Read the model definition and answer for the solid it produces. Units are mm, in the model's axes. A direction names the side the tool comes from. Coordinates: 2 decimals unless noted, no trailing zeros. Loops run counter-clockwise (first coordinate to the right, second up) from the corner with the lowest first, then second, coordinate; pieces in that order, holes last.
from build123d import *

# Parameters (mm, degrees)
SKETCH1_R               = 23
BOSS_EXTRUDE3_DEPTH     = 10
SKETCH3_R               = 23
SKETCH3_R_2             = 13
CUT_EXTRUDE1_DEPTH      = 4
SKETCH4_R               = 1.725
SKETCH4_R_2             = 2.725
CUT_EXTRUDE2_DEPTH      = 35.029399054
SKETCH5_R               = 6.5
CUT_EXTRUDE3_DEPTH      = 5
SKETCH6_R               = 2.725
CUT_EXTRUDE4_DEPTH      = 35.029399054
CUT_EXTRUDE5_DEPTH      = 34.075670817
CUT_EXTRUDE5_DEPTH_BACK = 4
FILLET1_R               = 2


with BuildPart() as part:
    # Sketch1 → Boss-Extrude3 (new body)
    with BuildSketch(Plane.XY):
        Circle(SKETCH1_R)
    extrude(amount=BOSS_EXTRUDE3_DEPTH)

    # Sketch3 → Cut-Extrude1 (cut)
    with BuildSketch(Plane(origin=(0, 0, 0), x_dir=(-1, 0, 0), z_dir=(0, 0, -1))):
        Circle(SKETCH3_R)
        Circle(SKETCH3_R_2, mode=Mode.SUBTRACT)
    extrude(amount=-CUT_EXTRUDE1_DEPTH, mode=Mode.SUBTRACT)

    # Sketch4 → Cut-Extrude2 (cut, through all)
    with BuildSketch(Plane(origin=(0, 0, 0), x_dir=(-1, 0, 0), z_dir=(0, 0, -1))):
        with Locations((-7.071067812, -7.071067812)):
            Circle(SKETCH4_R)
        with Locations((7.071067812, 7.071067812)):
            Circle(SKETCH4_R)
        Circle(SKETCH4_R_2)
        with Locations((-7.071067812, 7.071067812)):
            Circle(SKETCH4_R)
        with Locations((7.071067812, -7.071067812)):
            Circle(SKETCH4_R)
    extrude(amount=-CUT_EXTRUDE2_DEPTH, mode=Mode.SUBTRACT)

    # Sketch5 → Cut-Extrude3 (cut)
    with BuildSketch(Plane.XY.offset(10)):
        Circle(SKETCH5_R)
        Polygon((-7.92281451, 10.249829766), (-10.249829766, 7.92281451), (-9.398083068, 4.744052556), (-6.219321113, 3.892305858), (-3.892305858, 6.219321113), (-4.744052556, 9.398083068), align=None)
        Polygon((9.398083068, -4.744052556), (6.219321113, -3.892305858), (3.892305858, -6.219321113), (4.744052556, -9.398083068), (7.92281451, -10.249829766), (10.249829766, -7.92281451), align=None)
        Polygon((-3.892305858, -6.219321113), (-6.219321113, -3.892305858), (-9.398083068, -4.744052556), (-10.249829766, -7.92281451), (-7.92281451, -10.249829766), (-4.744052556, -9.398083068), align=None)
        Polygon((9.398083068, 4.744052556), (10.249829766, 7.92281451), (7.92281451, 10.249829766), (4.744052556, 9.398083068), (3.892305858, 6.219321113), (6.219321113, 3.892305858), align=None)
    extrude(amount=-CUT_EXTRUDE3_DEPTH, mode=Mode.SUBTRACT)

    # Sketch6 → Cut-Extrude4 (cut, through all)
    with BuildSketch(Plane.XY.offset(10)):
        with Locations((0, 16.5)):
            Circle(SKETCH6_R)
        with Locations((0, -16.5)):
            Circle(SKETCH6_R)
    extrude(amount=-CUT_EXTRUDE4_DEPTH, mode=Mode.SUBTRACT)

    # Sketch7 → Cut-Extrude5 (cut, two sides: drawn at the far end of the back side and taken through both)
    with BuildSketch(Plane(origin=(0, 0, 4), x_dir=(-1, 0, 0), z_dir=(0, 0, -1)).offset(-CUT_EXTRUDE5_DEPTH_BACK)):
        Polygon((4.734272207, 16.5), (2.367136104, 20.6), (-2.367136104, 20.6), (-4.734272207, 16.5), (-2.367136104, 12.4), (2.367136104, 12.4), align=None)
        Polygon((4.734272207, -16.5), (2.367136104, -12.4), (-2.367136104, -12.4), (-4.734272207, -16.5), (-2.367136104, -20.6), (2.367136104, -20.6), align=None)
    extrude(amount=CUT_EXTRUDE5_DEPTH + CUT_EXTRUDE5_DEPTH_BACK, mode=Mode.SUBTRACT)

    # Fillet1
    fillet1_edges = [part.edges().sort_by_distance(p)[0] for p in [
        (13, 0, 4),
        (-13, 0, 4),
        (-23, 0, 10),
        (-23, 0, 4),
    ]]
    fillet(fillet1_edges, radius=FILLET1_R)


solid = part.part
Q1. Determine the mould class of faces 4 (the face through (-1, 19.3, 8)), 5 (the face through (-5, -4.4, 10)) for opening direction X: +X half, -X half, draft (parallel to the pull), parting line (faces both ways), or undercut.
Findings below:
face 4: undercut
face 5: draft
Q2. A cutting plane is placed at A-A (y = 0). Give the vertices of the cut face in (x, z) (3 decimals).
Findings below:
outline: (-23, 6) arc R2 ccw to (-21, 4) - (-15, 4) arc R2 cw to (-13, 2) - (-13, 0) - (-2.725, 0) - (-2.725, 5) - (-6.5, 5) - (-6.5, 10) - (-21, 10) arc R2 ccw to (-23, 8) - close; (2.725, 0) - (13, 0) - (13, 2) arc R2 cw to (15, 4) - (21, 4) arc R2 ccw to (23, 6) - (23, 8) arc R2 ccw to (21, 10) - (6.5, 10) - (6.5, 5) - (2.725, 5) - close
Q3. Which of the six approach directions +Z, -Z, +X, -X, +Y, -Y give full straight-line access (tool end or side, diameter ignored) to faces 1 (the face through (3.534, -14.421, 5.834)), 2 (the face through (-4.324, -7.831, 7.535)), 3 (the face through (8.342, -5.905, 2.465))?
Findings below:
face 1: -Z
face 2: +Z
face 3: +Z, -Z
Q4. A cutting plane is placed at B-B (x = 0). Count the separate pieces of the cut face and the enclosed holes in it, then the cut area to 3 significant figures.
Findings below:
separate pieces: 4
enclosed holes: 0
area: 192 mm2
Q5. Straight lines are drawn through the part: probe 1 along X at (y, z) = (-7.5, 9.25); probe 2 along X at (y, z) = (7, 1.5); probe 3 along Y at (x, z) = (0, 8.6) (3 decimals). For each, find the intervals that lie inside material, in ascending order.
Findings below:
probe 1: x = -21.28 to -10.14, -4.24 to 4.24, 10.14 to 21.28
probe 2: x = -10.95 to -8.79, -5.35 to 5.35, 8.79 to 10.95
probe 3: y = -22.908 to -19.225, -13.775 to -6.5, 6.5 to 13.775, 19.225 to 22.908
Q6. Flat-ended cylindrical pins translate along their axes: pin 1 Ø4 at (y, z) = (-3, 3) entering from -X; pin 2 Ø4 at (x, z) = (1, 2.5) entering from +Y; pin 3 Ø6 at (y, z) = (-6.5, 5.5) entering from -X; pin 4 Ø3 at (x, y) = (7.07, -7.07) entering from -Z. Find the tip coordinate at first contact, or state that the pin passes through.
Findings below:
pin 1: stops at x = -22.56
pin 2: stops at y = 22.3
pin 3: stops at x = -22.73
pin 4: passes through
